Verification items for this drawing (mm, ordinates from the low corner). A direction names the side the tool comes from. Round coordinates to 2 decimals unless told otherwise and drop trailing zeros. Write each loop counter-clockwise with the first axis right and the second up, starting at its lowest first coordinate (ties: lowest second). Pieces come first, ordered by that corner, then holes. Notation, with made-up numbers: (-17.5, -27.75) -> (22.5, -27.75) arc R13 cw to (22.5, -9.75) -> close; hole circle Ø7 at (78, 52). An arc over 180 degrees is marked (long way). Return JSON: item names as keys, results as strings. Group by question number.
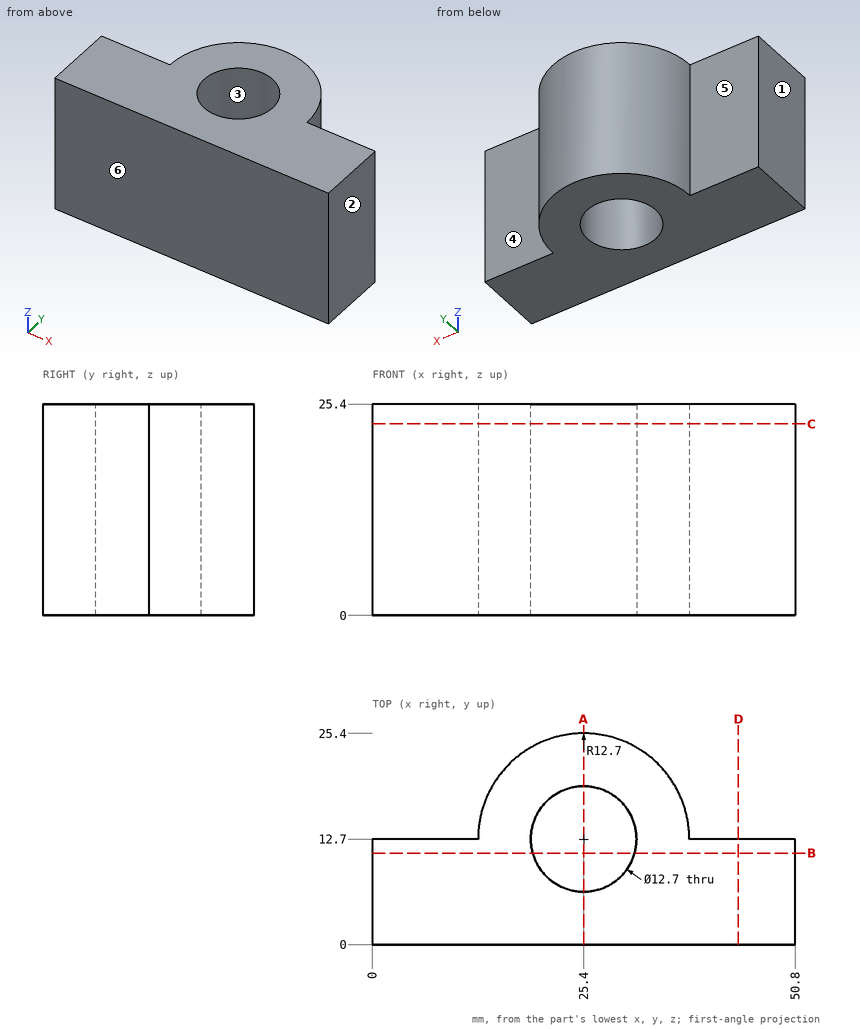
1) Tool access check on the marked faces 4, 5 and 6. Record the directions out of +Z, -Z, +X, -X, +Y, -Y that give a thin tool (end or side, any length) a straight path to the whole face; none if there is none.
2) Material ranges on probe 1 along Y at (x, z) = (25, 22); probe 2 along Y at (x, z) = (27, 8.75); probe 3 along X at (y, z) = (8, 13.5), recorded low to high. Write a range as [from, to].
3) Sectioned sample at B-B on y = 11. Enter the section's corners in (x, z), and give its area (3 significant figures).
4) Sectioned sample at A-A on x = 25.4. Enter the section's corners in (y, z), and give its area (3 significant figures).
5) Mould release check, pull along X, two halves, no side actions. Record for the marked faces 1, 2 and 3: +X half, -X half, draft (parallel to the pull), parting line (faces both ways), or undercut.
6) Go/stop test with flat-tipped pins: P1, Ø10, axis at y = 7, z = 14.5, coming from the -X side; P2, Ø2, axis at x = 43, y = 15, coming from the -Z side; P3, Ø12, axis at x = 39.5, z = 18.5, coming from the +Y side; P4, Ø12, axis at x = 32, z = 14, coming from the +Y side. Record where each tip stops, or that it passes through.
7) Sectioned sample at D-D on x = 44. Enter the section's corners in (y, z).
8) Sectioned sample at C-C on z = 23. Enter the section's corners in (x, y).
Evaluation:
{
 "1": {"face 4": "+Z, -Z, +X, +Y", "face 5": "+Z, -Z, -X, +Y", "face 6": "+Z, -Z, +X, -X, -Y"},
 "2": {"probe 1": "y = [0, 6.36], [19.04, 25.39]", "probe 2": "y = [0, 6.55], [18.85, 25.3]", "probe 3": "x = [0, 21.13], [29.67, 50.8]"},
 "3": {"outline": "(0, 0) -> (19.28, 0) -> (19.28, 25.4) -> (0, 25.4) -> close; (31.52, 0) -> (50.8, 0) -> (50.8, 25.4) -> (31.52, 25.4) -> close", "area": "980 mm2"},
 "4": {"outline": "(0, 0) -> (6.35, 0) -> (6.35, 25.4) -> (0, 25.4) -> close; (19.05, 0) -> (25.4, 0) -> (25.4, 25.4) -> (19.05, 25.4) -> close", "area": "323 mm2"},
 "5": {"face 1": "-X half", "face 2": "+X half", "face 3": "undercut"},
 "6": {"P1": "stops at x = 0", "P2": "passes through", "P3": "stops at y = 22.48", "P4": "stops at y = 25.39"},
 "7": {"outline": "(0, 0) -> (12.7, 0) -> (12.7, 25.4) -> (0, 25.4) -> close"},
 "8": {"outline": "(0, 0) -> (50.8, 0) -> (50.8, 12.7) -> (38.1, 12.7) arc R12.7 ccw to (12.7, 12.7) -> (0, 12.7) -> close; hole circle Ø12.7 at (25.4, 12.7)"}
}
